from build123d import *

# Parameters (mm, degrees)
SKETCH1_W              = 304.8
SKETCH1_H              = 152.4
SKETCH1_R              = 3.175
SKETCH1_R_2            = 2.794
BOARD_DEPTH            = 2.54
SKETCH3_W              = 53.086
SKETCH3_H              = 11.43
D25TOCOMPUTER_DEPTH    = 12.7
SKETCH5_W              = 39.116
SKETCH5_H              = 11.43
D15TOMOTOR_BRAKE_DEPTH = 12.7
SKETCH9_W              = 8.89
SKETCH9_H              = 45.72
SKETCH9_R              = 2.286
MOTORS_BRAKES_DEPTH    = 6.35
SKETCH10_W             = 12.7
SKETCH10_H             = 152.4
SKETCH10_R             = 3.175
PLATEDEDGE_DEPTH       = 0.0254
SKETCH11_W             = 45.72
SKETCH11_H             = 8.89
SKETCH11_R             = 2.286
HVIN_24VIN_5VIN_DEPTH  = 6.4516


with BuildPart() as part:
    # Sketch1 → Board (new body)
    with BuildSketch(Plane(origin=(0, 0, 0), x_dir=(1, 0, 0), z_dir=(0, 1, 0))):
        with Locations((152.4, 76.2)):
            Rectangle(SKETCH1_W, SKETCH1_H)
        with Locations(Location((298.731278283, 76.2, 0), (0, 0, 270))):
            Circle(SKETCH1_R, mode=Mode.SUBTRACT)
        with Locations(Location((298.731278283, 133.35, 0), (0, 0, 270))):
            Circle(SKETCH1_R, mode=Mode.SUBTRACT)
        with Locations(Location((298.731278283, 19.05, 0), (0, 0, 90))):
            Circle(SKETCH1_R, mode=Mode.SUBTRACT)
        with Locations(Location((6.068721717, 19.05, 0), (0, 0, 270))):
            Circle(SKETCH1_R, mode=Mode.SUBTRACT)
        with Locations(Location((6.068721717, 76.2, 0), (0, 0, 90))):
            Circle(SKETCH1_R, mode=Mode.SUBTRACT)
        with Locations(Location((6.068721717, 133.35, 0), (0, 0, 90))):
            Circle(SKETCH1_R, mode=Mode.SUBTRACT)
        with Locations(Location((63.5, 9.525, 0), (0, 0, 270))):
            Circle(SKETCH1_R_2, mode=Mode.SUBTRACT)
        with Locations(Location((63.5, 97.917, 0), (0, 0, 270))):
            Circle(SKETCH1_R_2, mode=Mode.SUBTRACT)
        with Locations(Location((146.05, 97.917, 0), (0, 0, 270))):
            Circle(SKETCH1_R_2, mode=Mode.SUBTRACT)
        with Locations(Location((146.05, 9.525, 0), (0, 0, 270))):
            Circle(SKETCH1_R_2, mode=Mode.SUBTRACT)
    extrude(amount=BOARD_DEPTH)

    # Sketch3 → D25toComputer (add)
    with BuildSketch(Plane(origin=(0, 2.54, 0), x_dir=(-1, 0, 0), z_dir=(0, 1, 0))):
        with Locations((-75.767610713, -144.145)):
            Rectangle(SKETCH3_W, SKETCH3_H)
    extrude(amount=D25TOCOMPUTER_DEPTH)

    # Sketch5 → D15toMotor/Brake (add)
    with BuildSketch(Plane(origin=(0, 2.54, 0), x_dir=(-1, 0, 0), z_dir=(0, 1, 0))):
        with Locations((-177.038519959, -144.145)):
            Rectangle(SKETCH5_W, SKETCH5_H)
        with Locations((-223.715302991, -144.145)):
            Rectangle(SKETCH5_W, SKETCH5_H)
    extrude(amount=D15TOMOTOR_BRAKE_DEPTH)

    # Sketch9 → Motors/Brakes (add)
    # profile 1 of 2: a face of its own
    with BuildSketch(Plane(origin=(0, 2.54, 0), x_dir=(-1, 0, 0), z_dir=(0, 1, 0))):
        with Locations((-251.635702832, -86.062744457)):
            Rectangle(SKETCH9_W, SKETCH9_H)
        with Locations(Location((-251.635702832, -73.524162022, 0), (0, 0, 90))):
            Circle(SKETCH9_R, mode=Mode.SUBTRACT)
        with Locations(Location((-251.635702832, -67.174162022, 0), (0, 0, 90))):
            Circle(SKETCH9_R, mode=Mode.SUBTRACT)
        with Locations(Location((-251.635702832, -86.224162022, 0), (0, 0, 90))):
            Circle(SKETCH9_R, mode=Mode.SUBTRACT)
        with Locations(Location((-251.635702832, -79.874162022, 0), (0, 0, 90))):
            Circle(SKETCH9_R, mode=Mode.SUBTRACT)
        with Locations(Location((-251.635702832, -98.924162022, 0), (0, 0, 90))):
            Circle(SKETCH9_R, mode=Mode.SUBTRACT)
        with Locations(Location((-251.635702832, -92.574162022, 0), (0, 0, 90))):
            Circle(SKETCH9_R, mode=Mode.SUBTRACT)
        with Locations(Location((-251.635702832, -105.274162022, 0), (0, 0, 90))):
            Circle(SKETCH9_R, mode=Mode.SUBTRACT)
    # profile 2 of 2: a face of its own
    with BuildSketch(Plane(origin=(0, 2.54, 0), x_dir=(-1, 0, 0), z_dir=(0, 1, 0))):
        with Locations((-232.585702832, -86.062744457)):
            Rectangle(SKETCH9_W, SKETCH9_H)
        with Locations(Location((-232.585702832, -79.874162022, 0), (0, 0, 90))):
            Circle(SKETCH9_R, mode=Mode.SUBTRACT)
        with Locations(Location((-232.585702832, -67.174162022, 0), (0, 0, 90))):
            Circle(SKETCH9_R, mode=Mode.SUBTRACT)
        with Locations(Location((-232.585702832, -98.924162022, 0), (0, 0, 90))):
            Circle(SKETCH9_R, mode=Mode.SUBTRACT)
        with Locations(Location((-232.585702832, -105.274162022, 0), (0, 0, 90))):
            Circle(SKETCH9_R, mode=Mode.SUBTRACT)
        with Locations(Location((-232.585702832, -73.524162022, 0), (0, 0, 90))):
            Circle(SKETCH9_R, mode=Mode.SUBTRACT)
        with Locations(Location((-232.585702832, -86.224162022, 0), (0, 0, 90))):
            Circle(SKETCH9_R, mode=Mode.SUBTRACT)
        with Locations(Location((-232.585702832, -92.574162022, 0), (0, 0, 90))):
            Circle(SKETCH9_R, mode=Mode.SUBTRACT)
    extrude(amount=MOTORS_BRAKES_DEPTH)

    # Sketch10 → platedEdge (add)
    # profile 1 of 2: a face of its own
    with BuildSketch(Plane(origin=(0, 2.54, 0), x_dir=(-1, 0, 0), z_dir=(0, 1, 0))):
        with Locations((-298.45, -76.2)):
            Rectangle(SKETCH10_W, SKETCH10_H)
        with Locations(Location((-298.731278283, -133.35, 0), (0, 0, 90))):
            Circle(SKETCH10_R, mode=Mode.SUBTRACT)
        with Locations(Location((-298.731278283, -76.2, 0), (0, 0, 90))):
            Circle(SKETCH10_R, mode=Mode.SUBTRACT)
        with Locations(Location((-298.731278283, -19.05, 0), (0, 0, 270))):
            Circle(SKETCH10_R, mode=Mode.SUBTRACT)
    # profile 2 of 2: a face of its own
    with BuildSketch(Plane(origin=(0, 2.54, 0), x_dir=(-1, 0, 0), z_dir=(0, 1, 0))):
        with Locations((-6.35, -76.2)):
            Rectangle(SKETCH10_W, SKETCH10_H)
        with Locations(Location((-6.068721717, -19.05, 0), (0, 0, 90))):
            Circle(SKETCH10_R, mode=Mode.SUBTRACT)
        with Locations(Location((-6.068721717, -76.2, 0), (0, 0, 270))):
            Circle(SKETCH10_R, mode=Mode.SUBTRACT)
        with Locations(Location((-6.068721717, -133.35, 0), (0, 0, 270))):
            Circle(SKETCH10_R, mode=Mode.SUBTRACT)
    extrude(amount=PLATEDEDGE_DEPTH)

    # Sketch11 → HVin/24Vin/5Vin (add)
    with BuildSketch(Plane(origin=(0, 2.54, 0), x_dir=(-1, 0, 0), z_dir=(0, 1, 0))):
        with Locations((-247.144556465, -38.354996588)):
            Rectangle(SKETCH11_W, SKETCH11_H)
        with Locations(Location((-259.683138901, -38.354996588, 0), (0, 0, 90))):
            Circle(SKETCH11_R, mode=Mode.SUBTRACT)
        with Locations(Location((-227.933138901, -38.354996588, 0), (0, 0, 90))):
            Circle(SKETCH11_R, mode=Mode.SUBTRACT)
        with Locations(Location((-253.333138901, -38.354996588, 0), (0, 0, 90))):
            Circle(SKETCH11_R, mode=Mode.SUBTRACT)
        with Locations(Location((-234.283138901, -38.354996588, 0), (0, 0, 90))):
            Circle(SKETCH11_R, mode=Mode.SUBTRACT)
        with Locations(Location((-246.983138901, -38.354996588, 0), (0, 0, 90))):
            Circle(SKETCH11_R, mode=Mode.SUBTRACT)
        with Locations(Location((-266.033138901, -38.354996588, 0), (0, 0, 90))):
            Circle(SKETCH11_R, mode=Mode.SUBTRACT)
        with Locations(Location((-240.633138901, -38.354996588, 0), (0, 0, 90))):
            Circle(SKETCH11_R, mode=Mode.SUBTRACT)
    extrude(amount=HVIN_24VIN_5VIN_DEPTH)


solid = part.part
CAD build for the part. Positions are in the model's coordinates, mm. A direction names the side the tool comes from. Coordinates: 2 decimals unless noted, no trailing zeros. Write each loop counter-clockwise with the first axis right and the second up, starting at its lowest first coordinate (ties: lowest second). Pieces come first, ordered by that corner, then holes. Notation, with made-up numbers: (64, 70) - (92, 70) arc R19 cw to (92, 77) - close; hole circle Ø10 at (12, 69.25). An arc over 180 degrees is marked (long way). Use a Markdown table: item, result. Add a question column.
Item 1: Mould opens along Z. For faces 1 (the face through (76, 9, -149.86)), 2 (the face through (228.141, 6, -86)), 3 (the face through (7.02, 1.26, -16.02)), 4 (the face through (157.481, 9, -144)) say: pulls with the +Z half, pulls with the -Z half, needs draft (parallel to the pull), parting line crosses it, or undercut.
Item 2: 3-axis set-ups, long thin cutter, end or side, ignore diameter. For faces 5 (the face through (224.285, 6, -38)), 6 (the face through (247, 8.992, -35)), 7 (the face through (270.005, 6, -38)): which of +Z, -Z, +X, -X, +Y, -Y reach the whole face in a straight line?
Item 3: Band-saw the part on B-B, the plane z = -133.35. Give the number of separate pieces and of enclosed holes in the cut face, and give its area (3 significant figures).
Item 4: Drill centre lines: L1, parallel to X at y = 1.4, z = -133.35; L2, parallel to Z at x = 146.05, y = 1.4; L3, parallel to Z at x = 238, y = 5.75. Where is each one in solid material? Low to high. Write a range as from..to.
Item 5: Band-saw the part on A-A, the plane x = 63.5. Give the cut face in (y, z).
Item 6: Flat gauge pins, fed straight in: pin 1 (2.5 mm diameter, centred on x = 250.5, z = -81, fed in from +Y); pin 2 (5 mm diameter, centred on x = 230.5, z = -129.5, fed in from -Y); pin 3 (6.5 mm diameter, centred on x = 176.5, y = 9, fed in from +Z); pin 4 (1.5 mm diameter, centred on x = 192.5, y = 9, fed in from -Z). Where does each tip first touch, or does it go through?
Numbers:
| question | item | result |
|---|---|---|
| 1 | face 1 | pulls with the -Z half |
| 1 | face 2 | undercut |
| 1 | face 3 | undercut |
| 1 | face 4 | needs draft |
| 2 | face 5 | +Z, -X, +Y |
| 2 | face 6 | +Z, +X, -X, +Y |
| 2 | face 7 | +Z, -Z, +X, +Y |
| 3 | separate pieces | 3 |
| 3 | enclosed holes | 0 |
| 3 | area | 742 mm2 |
| 4 | L1 | 0..2.89, 9.24..295.56, 301.91..304.8 |
| 4 | L2 | -152.4..-100.71, -95.12..-12.32, -6.73..0 |
| 4 | L3 | -149.86..-138.43, -42.8..-33.91 |
| 5 | outline | (0, -152.4) - (2.54, -152.4) - (2.54, -149.86) - (15.24, -149.86) - (15.24, -138.43) - (2.54, -138.43) - (2.54, -100.71) - (0, -100.71) - close; (0, -95.12) - (2.54, -95.12) - (2.54, -12.32) - (0, -12.32) - close; (0, -6.73) - (2.54, -6.73) - (2.54, 0) - (0, 0) - close |
| 6 | pin 1 | y = 8.89 |
| 6 | pin 2 | y = 0 |
| 6 | pin 3 | z = -138.43 |
| 6 | pin 4 | z = -149.86 |
